The listing builds one solid part. Answer for the finished solid, in the listing's coordinates (mm). Face numbers are marked on the shaded views. A direction names the side the tool comes from. Give positions to 0.01 mm unless a question says otherwise; leave off trailing zeros. Order: outer loops, then holes, each group sorted by start corner. A loop starts at its lowest first (then second) coordinate and runs counter-clockwise, first axis right, second up. Notation, with made-up numbers: (-14.75, 53) - (14.25, 53) arc R18 ccw to (14.25, 63) - close; hole circle Ø9 at (69.5, 21). An arc over 180 degrees is marked (long way). Use CSV: the item, a comma, the result in double quotes.
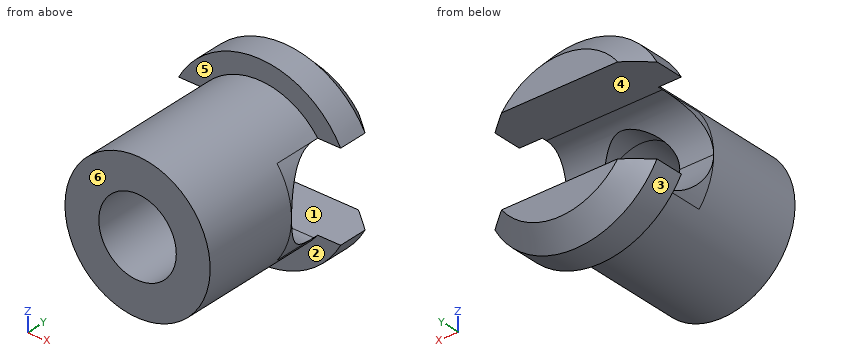
```python
from build123d import *
from build123d.topology import SkipClean

# Parameters (mm, degrees)
SKETCH2_R               = 4
CUT_EXTRUDE1_DEPTH      = 25.093567606
CUT_EXTRUDE2_DEPTH      = 25.093567606
CUT_EXTRUDE2_DEPTH_BACK = 25.093567606
SKETCH3_W               = 9
SKETCH3_H               = 10
FILLET1_START           = 10
FILLET1_OUTLINE_R       = 4
FILLET1_DEPTH           = 4.5000001
FILLET1_START_2         = -7.500000249
FILLET1_2_DEPTH         = 15.000000249


with BuildPart() as part:
    # Sketch1 → Revolve1 (revolve)
    with BuildSketch(Plane.XY, mode=Mode.PRIVATE) as revolve1_sk:
        Polygon((0, 0), (7.5, 0), (7.5, 15), (9.5, 15), (9.5, 18), (7.5, 20), (0, 20), align=None)
    revolve(revolve1_sk.sketch.rotate(Axis((0, 20, 0), (0, -1, 0)), 180), axis=Axis((0, 20, 0), (0, -1, 0)))

    # Sketch2 → Cut-Extrude1 (cut, through all)
    with BuildSketch(Plane.XZ):
        Circle(SKETCH2_R)
    extrude(amount=-CUT_EXTRUDE1_DEPTH, mode=Mode.SUBTRACT)

    # Sketch3 → Cut-Extrude2 (cut, two sides: drawn at the far end of the back side and taken through both)
    with BuildSketch(Plane(origin=(0, 0, 0), x_dir=(0, 0, -1), z_dir=(1, 0, 0)).offset(-CUT_EXTRUDE2_DEPTH_BACK)):
        with Locations((0, 15)):
            Rectangle(SKETCH3_W, SKETCH3_H)
    extrude(amount=CUT_EXTRUDE2_DEPTH + CUT_EXTRUDE2_DEPTH_BACK, mode=Mode.SUBTRACT)

    # Fillet1: read off the stored shape, not the designer's step
    # Fillet1 outline → Fillet1 (add)
    with SkipClean():  # the faces are left unmerged after this step: merging them gives an invalid solid
        with BuildSketch(Plane(origin=(0, 0, 0), x_dir=(1, 0, 0), z_dir=(0, 1, 0)).offset(FILLET1_START)):
            with BuildLine():
                ThreePointArc((6, -4.5), (7.5, 0), (6, 4.5))
                Line((6, 4.5), (-6, 4.5))
                ThreePointArc((-6, 4.5), (-7.5, 0), (-6, -4.5))
                Line((-6, -4.5), (6, -4.5))
            make_face()
            Circle(FILLET1_OUTLINE_R, mode=Mode.SUBTRACT)
        extrude(amount=FILLET1_DEPTH)

    # Fillet1 2 outline → Fillet1 2 (cut)
    with SkipClean():  # the faces are left unmerged after this step: merging them gives an invalid solid
        with BuildSketch(Plane.YZ.offset(FILLET1_START_2)):
            with BuildLine():
                ThreePointArc((10, 0), (11.318019485, -3.181980515), (14.5, -4.5))
                Line((14.5, -4.5), (14.5, 4.5))
                ThreePointArc((14.5, 4.5), (11.318019485, 3.181980515), (10, 0))
            make_face()
        extrude(amount=FILLET1_2_DEPTH, mode=Mode.SUBTRACT)


solid = part.part
```
Item 1: The part is cut by section D-D (y = 3.75). Give the vertices of the cut face in (x, z), and give its area (3 significant figures).
Taken from the geometry:
outline,"circle Ø15 at (0, 0); hole circle Ø8 at (0, 0)"
area,"126 mm^2"
Item 2: Each of these flat-tipped pins is pushed along its axis until it touches: pin 1 (2.5 mm diameter, centred on x = 4, z = -8, fed in from -Y); pin 2 (2.5 mm diameter, centred on x = -3, y = 17, fed in from +Z); pin 3 (2 mm diameter, centred on x = -3, y = 4.5, fed in from +Z). Where does it stop, or does it pass through?
Taken from the geometry:
pin 1,"y = 15"
pin 2,"z = 9.34"
pin 3,"z = 7.23"
Item 3: The part is cut by section C-C (y = 10.75). Give the vertices of the cut face in (x, z).
Taken from the geometry:
outline,"(-7.08, -2.49) arc R7.5 ccw to (7.08, -2.49) - (3.13, -2.49) arc R4 cw to (-3.13, -2.49) - close; (-7.08, 2.49) - (-3.13, 2.49) arc R4 cw to (3.13, 2.49) - (7.08, 2.49) arc R7.5 ccw to start"
Item 4: Find the intervals of material crossed by line 1 along Z through (x, y) = (0, 6.5); line 2 along X through (y, z) = (3.5, -6); line 3 along Z through (x, y) = (0.75, 3), in increasing order.
Taken from the geometry:
line 1,"-7.5 to -4, 4 to 7.5"
line 2,"-4.5 to 4.5"
line 3,"-7.46 to -3.93, 3.93 to 7.46"
Item 5: The part is cut by section A-A (x = 0). Give the vertices of the cut face in (y, z), and give its area (3 significant figures).
Taken from the geometry:
outline,"(0, -7.5) - (15, -7.5) - (15, -9.5) - (18, -9.5) - (20, -7.5) - (20, -4.5) - (14.5, -4.5) arc R4.5 cw to (12.44, -4) - (0, -4) - close; (0, 4) - (12.44, 4) arc R4.5 cw to (14.5, 4.5) - (20, 4.5) - (20, 7.5) - (18, 9.5) - (15, 9.5) - (15, 7.5) - (0, 7.5) - close"
area,"149 mm^2"
Item 6: Which of the six approach directions +Z, -Z, +X, -X, +Y, -Y give full straight-line access (tool end or side, diameter ignored) to the marked faces 4, 5 and 6?
Taken from the geometry:
face 4,"+X, -X, +Y"
face 5,"+Z, -Y"
face 6,"+Z, -Z, +X, -X, -Y"
Item 7: The part is cut by section B-B (z = -0.5). Give the vertices of the cut face in (x, y).
Taken from the geometry:
outline,"(-7.48, 0) - (-3.97, 0) - (-3.97, 10.03) - (-7.48, 10.03) - close; (3.97, 0) - (7.48, 0) - (7.48, 10.03) - (3.97, 10.03) - close"
Item 8: The mould has two halves that part along Z. Classify the marked faces 1, 2 and 3: +Z half, -Z half, draft (parallel to the pull), parting line (faces both ways), or undercut.
Taken from the geometry:
face 1,"undercut"
face 2,"draft"
face 3,"-Z half"
